Design review of the part built by this model. Coordinates are the model's own, in mm. A direction names the side the tool comes from. Round coordinates to 2 decimals unless told otherwise and drop trailing zeros. Loops run counter-clockwise (first coordinate to the right, second up) from the corner with the lowest first, then second, coordinate; pieces in that order, holes last. Notation, with made-up numbers: (-0.75, 0.5) - (6.25, 0.5) arc R15 cw to (6.25, 23.5) - close; hole circle Ø10 at (39.25, 8.25). An arc over 180 degrees is marked (long way). Use one line per item in the form item = value. Start each with the question number.
(1) We need section B-B, the plane x = -15. Write out the cut boundary in (y, z), then the cut area to 3 significant figures.
(2) We need section D-D, the plane y = 14. Write out the cut boundary in (x, z), then the cut area to 3 significant figures.
(3) For pin 1 (2.5 mm diameter, centred on x = -15, y = -24, fed in from +Z); pin 2 (1.6 mm diameter, centred on x = -15, y = 24, fed in from +Z), all flat-tipped, find the tip position at first contact; note any pin that passes through.
(4) Wall thickness on probe 1 along Y at (x, z) = (15, 0.7); probe 2 along X at (y, z) = (-5.5, 0.4); probe 3 along X at (y, z) = (11, 0.9): over which ranges is each line inside the solid? List them lowest first. Write a range as [from, to].
(5) We need section A-A, the plane z = 0.7. Write out the cut boundary in (x, y), then the cut area to 3 significant figures.
(6) We need section C-C, the plane x = 0. Write out the cut boundary in (y, z).
(7) Machinability: for faces 3 (the flat face through (-16, 25, 1)), 4 (the flat face through (-16, -25, 1)), 5 (the flat face through (16, -26, 1)), which of the approach directions +Z, -Z, +X, -X, +Y, -Y give a long, thin tool a straight path to every point of the face, cutting with its end or side? Answer none if there is none.
(8) The part is to be moulded in two halves that separate along X. For faces 1 (the flat face through (16, 25, 1)), 2 (the cylindrical face through (17.01, 27.06, 0.49)), say which applies: released by +X, released by -X, zero draft, split by the parting line, or undercut.
from build123d import *

# Parameters (mm, degrees)
SKETCH_1_R          = 26.5
EXTRUDE_2_DEPTH     = 1.7
EXTRUDE_3_DEPTH     = 1
SKETCH_4_R          = 1
CUT_EXTRUDE_1_DEPTH = 1


with BuildPart() as part:
    # Эскиз1 → Бобышка-Вытянуть2 (new body)
    with BuildSketch(Plane.XY):
        Circle(SKETCH_1_R)
    extrude(amount=EXTRUDE_2_DEPTH)

    # Эскиз3 → Бобышка-Вытянуть3 (add)
    with BuildSketch(Plane.XY):
        with BuildLine():
            Line((0, 6.907283337), (-11.895602995, 25.940248128))
            ThreePointArc((-11.895602995, 25.940248128), (-16.940248128, 27.104397005), (-18.104397005, 22.059751872))
            Line((-18.104397005, 22.059751872), (-4.317052086, 0))
            Line((-4.317052086, 0), (0, 6.907283337))
        make_face()
        with BuildLine():
            Line((11.895602995, 25.940248128), (0, 6.907283337))
            Line((0, 6.907283337), (4.317052086, 0))
            Line((4.317052086, 0), (18.104397005, 22.059751872))
            ThreePointArc((18.104397005, 22.059751872), (16.940248128, 27.104397005), (11.895602995, 25.940248128))
        make_face()
        with BuildLine():
            Line((0, -6.907283337), (-4.317052086, 0))
            Line((-4.317052086, 0), (-18.104397005, -22.059751872))
            ThreePointArc((-18.104397005, -22.059751872), (-16.940248128, -27.104397005), (-11.895602995, -25.940248128))
            Line((-11.895602995, -25.940248128), (0, -6.907283337))
        make_face()
        with BuildLine():
            Line((18.104397005, -22.059751872), (4.317052086, 0))
            Line((4.317052086, 0), (0, -6.907283337))
            Line((0, -6.907283337), (11.895602995, -25.940248128))
            ThreePointArc((11.895602995, -25.940248128), (16.940248128, -27.104397005), (18.104397005, -22.059751872))
        make_face()
    extrude(amount=EXTRUDE_3_DEPTH)

    # Эскиз4 → Вырез-Вытянуть1 (cut)
    with BuildSketch(Plane.XY.offset(1)):
        with Locations((-15, 24)):
            Circle(SKETCH_4_R)
        with Locations((15, 24)):
            Circle(SKETCH_4_R)
        with Locations((15, -24)):
            Circle(SKETCH_4_R)
        with Locations((-15, -24)):
            Circle(SKETCH_4_R)
    extrude(amount=-CUT_EXTRUDE_1_DEPTH, mode=Mode.SUBTRACT)


solid = part.part
Data:
q1.outline = (-27.66, 0) - (-25, 0) - (-25, 1) - (-27.66, 1) - close; (-23, 0) - (23, 0) - (23, 1) - (21.85, 1) - (21.85, 1.7) - (-21.85, 1.7) - (-21.85, 1) - (-23, 1) - close; (25, 0) - (27.66, 0) - (27.66, 1) - (25, 1) - close
q1.area = 81.9 mm^2
q2.outline = (-22.5, 0) - (22.5, 0) - (22.5, 1.7) - (-22.5, 1.7) - close
q2.area = 76.5 mm^2
q3.pin_1 = 1
q3.pin_2 = through
q4.probe_1 = [-27.66, -25], [-23, 23], [25, 27.66]
q4.probe_2 = [-25.92, 25.92]
q4.probe_3 = [-24.11, 24.11]
q5.outline = (-18.1, -22.06) arc R3.66 ccw to (-11.9, -25.94) - (-10.81, -24.2) arc R26.5 ccw to (10.81, -24.2) - (11.9, -25.94) arc R3.66 ccw to (18.1, -22.06) - (17.01, -20.32) arc R26.5 ccw to (17.01, 20.32) - (18.1, 22.06) arc R3.66 ccw to (11.9, 25.94) - (10.81, 24.2) arc R26.5 ccw to (-10.81, 24.2) - (-11.9, 25.94) arc R3.66 ccw to (-18.1, 22.06) - (-17.01, 20.32) arc R26.5 ccw to (-17.01, -20.32) - close; hole circle Ø2 at (-15, -24); hole circle Ø2 at (-15, 24); hole circle Ø2 at (15, -24); hole circle Ø2 at (15, 24)
q5.area = 2,330 mm^2
q6.outline = (-26.5, 0) - (26.5, 0) - (26.5, 1.7) - (-26.5, 1.7) - close
q7.face_3 = +Z, -X, +Y
q7.face_4 = +Z, -X, -Y
q7.face_5 = +Z, +X, -Y
q8.face_1 = zero draft
q8.face_2 = undercut
